Read the model definition and answer for the solid it produces. Units are mm, in the model's axes. Face numbers are marked on the shaded views. A direction names the side the tool comes from. Give positions to 0.01 mm unless a question says otherwise; leave off trailing zeros. Write each loop counter-clockwise with the first axis right and the second up, starting at its lowest first coordinate (ties: lowest second). Pieces come first, ordered by that corner, then holes. Notation, with made-up numbers: (9, 22) -> (42, 22) arc R23 ccw to (42, 61) -> close; hole circle Ø10 at (-13, 39.5). An arc over 180 degrees is marked (long way). Put each result on its own line as item: value. Start each with the question number.
from build123d import *

# Parameters (mm, degrees)
SKETCH1_W           = 130
SKETCH1_H           = 30
BOSS_EXTRUDE1_DEPTH = 5
BOSS_EXTRUDE3_DEPTH = 1.8
SKETCH6_W           = 40
SKETCH6_H           = 25
CUT_EXTRUDE2_DEPTH  = 2
SKETCH5_R           = 1.35
CUT_EXTRUDE3_DEPTH  = 6
SKETCH8_W           = 5
SKETCH8_H           = 30
BOSS_EXTRUDE4_DEPTH = 50
SKETCH9_R           = 10
CUT_EXTRUDE4_DEPTH  = 5
SKETCH10_W          = 30
SKETCH10_H          = 11.1
BOSS_EXTRUDE5_DEPTH = 30
SKETCH11_W          = 3.4
SKETCH11_H          = 30
CUT_EXTRUDE5_DEPTH  = 7
CUT_EXTRUDE6_REACH  = 173.828
SKETCH12_R          = 2.05
CUT_EXTRUDE7_DEPTH  = 5
SKETCH14_W          = 17.3
SKETCH14_H          = 30
CUT_EXTRUDE8_DEPTH  = 2
SKETCH15_W          = 2
SKETCH15_H          = 3
CUT_EXTRUDE9_DEPTH  = 15
FILLET1_START       = -1
FILLET1_DEPTH       = 161
FILLET1_START_2     = 5
FILLET1_2_DEPTH     = 155
FILLET3_R           = 1
FILLET6_R           = 1


with BuildPart() as part:
    # Sketch1 → Boss-Extrude1 (new body)
    with BuildSketch(Plane(origin=(0, 0, 0), x_dir=(1, 0, 0), z_dir=(0, 1, 0))):
        with Locations((65, -15)):
            Rectangle(SKETCH1_W, SKETCH1_H)
    extrude(amount=BOSS_EXTRUDE1_DEPTH)

    # Sketch4 → Boss-Extrude3 (add)
    with BuildSketch(Plane.XZ):
        Polygon((63.1, 25), (66.9, 25), (66.9, 17), (66.9, 16.95), (67.95, 16.95), (74.95, 16.95), (74.95, 13.15), (66.95, 13.15), (66.9, 13.15), (66.9, 12.1), (66.9, 5.1), (63.1, 5.1), (63.1, 13.1), (63.1, 13.15), (62.05, 13.15), (55.05, 13.15), (55.05, 16.95), (63.05, 16.95), (63.1, 16.95), (63.1, 18), align=None)
    extrude(amount=BOSS_EXTRUDE3_DEPTH)

    # Sketch6 → Cut-Extrude2 (cut)
    with BuildSketch(Plane(origin=(0, 5, 0), x_dir=(1, 0, 0), z_dir=(0, 1, 0))):
        with Locations((65, -15)):
            Rectangle(SKETCH6_W, SKETCH6_H)
    extrude(amount=-CUT_EXTRUDE2_DEPTH, mode=Mode.SUBTRACT)

    # Sketch5 → Cut-Extrude3 (cut)
    with BuildSketch(Plane.XZ.offset(1.8)):
        with Locations(Location((65, 23, 0), (0, 0, 270))):
            Circle(SKETCH5_R)
        with Locations(Location((73, 15, 0), (0, 0, 270))):
            Circle(SKETCH5_R)
        with Locations(Location((57, 15, 0), (0, 0, 270))):
            Circle(SKETCH5_R)
        with Locations(Location((65, 7, 0), (0, 0, 270))):
            Circle(SKETCH5_R)
    extrude(amount=-CUT_EXTRUDE3_DEPTH, mode=Mode.SUBTRACT)

    # Sketch8 → Boss-Extrude4 (add)
    with BuildSketch(Plane(origin=(0, 5, 0), x_dir=(1, 0, 0), z_dir=(0, 1, 0))):
        with Locations((2.5, -15)):
            Rectangle(SKETCH8_W, SKETCH8_H)
        with Locations((127.5, -15)):
            Rectangle(SKETCH8_W, SKETCH8_H)
    extrude(amount=BOSS_EXTRUDE4_DEPTH)

    # Sketch9 → Cut-Extrude4 (cut)
    with BuildSketch(Plane(origin=(130, 0, 0), x_dir=(0, 0, -1), z_dir=(1, 0, 0))):
        with Locations((-15, 40)):
            Circle(SKETCH9_R)
    extrude(amount=-CUT_EXTRUDE4_DEPTH, mode=Mode.SUBTRACT)

    # Sketch10 → Boss-Extrude5 (add)
    with BuildSketch(Plane(origin=(130, 0, 0), x_dir=(0, 0, -1), z_dir=(1, 0, 0))):
        with Locations((-15, 13.55)):
            Rectangle(SKETCH10_W, SKETCH10_H)
    extrude(amount=BOSS_EXTRUDE5_DEPTH)

    # Sketch11 → Cut-Extrude5 (cut)
    with BuildSketch(Plane(origin=(0, 19.1, 0), x_dir=(1, 0, 0), z_dir=(0, 1, 0))):
        with Locations((131.7, -15)):
            Rectangle(SKETCH11_W, SKETCH11_H)
        with Locations((152.4, -15)):
            Rectangle(SKETCH11_W, SKETCH11_H)
    extrude(amount=-CUT_EXTRUDE5_DEPTH, mode=Mode.SUBTRACT)

    # Cut-Extrude6: up to this face of the body (flat: up to its plane)
    cut_extrude6_end = Plane(part.part.faces().sort_by_distance((130, 12.623489255, 15))[0])
    # Sketch12 → Cut-Extrude6 (cut, up to the picked face)
    with BuildSketch(Plane(origin=(160, 0, 0), x_dir=(0, 0, -1), z_dir=(1, 0, 0)), mode=Mode.PRIVATE) as cut_extrude6_sk1:
        with Locations((-15, 16)):
            Circle(SKETCH12_R)
    cut_extrude6_tool1 = split(extrude(cut_extrude6_sk1.sketch, amount=-CUT_EXTRUDE6_REACH, mode=Mode.PRIVATE), bisect_by=cut_extrude6_end, keep=Keep.BOTH, mode=Mode.PRIVATE)
    # Sketch12 → Cut-Extrude6 (cut, up to the picked face)
    with BuildSketch(Plane(origin=(160, 0, 0), x_dir=(0, 0, -1), z_dir=(1, 0, 0)), mode=Mode.PRIVATE) as cut_extrude6_sk2:
        with Locations((-21, 16)):
            Circle(SKETCH12_R)
    cut_extrude6_tool2 = split(extrude(cut_extrude6_sk2.sketch, amount=-CUT_EXTRUDE6_REACH, mode=Mode.PRIVATE), bisect_by=cut_extrude6_end, keep=Keep.BOTH, mode=Mode.PRIVATE)
    # Sketch12 → Cut-Extrude6 (cut, up to the picked face)
    with BuildSketch(Plane(origin=(160, 0, 0), x_dir=(0, 0, -1), z_dir=(1, 0, 0)), mode=Mode.PRIVATE) as cut_extrude6_sk3:
        with Locations((-9, 16)):
            Circle(SKETCH12_R)
    cut_extrude6_tool3 = split(extrude(cut_extrude6_sk3.sketch, amount=-CUT_EXTRUDE6_REACH, mode=Mode.PRIVATE), bisect_by=cut_extrude6_end, keep=Keep.BOTH, mode=Mode.PRIVATE)
    add(cut_extrude6_tool1.solids().sort_by(Axis((160, 16, 15), (-1, 0, 0)))[0], mode=Mode.SUBTRACT)
    add(cut_extrude6_tool2.solids().sort_by(Axis((160, 16, 21), (-1, 0, 0)))[0], mode=Mode.SUBTRACT)
    add(cut_extrude6_tool3.solids().sort_by(Axis((160, 16, 9), (-1, 0, 0)))[0], mode=Mode.SUBTRACT)

    # Sketch13 → Cut-Extrude7 (cut)
    with BuildSketch(Plane.ZY):
        with BuildLine():
            Line((9, 40), (9, 55))
            Line((9, 55), (21, 55))
            Line((21, 55), (21, 40))
            ThreePointArc((21, 40), (15, 34), (9, 40))
        make_face()
    extrude(amount=-CUT_EXTRUDE7_DEPTH, mode=Mode.SUBTRACT)

    # Sketch14 → Cut-Extrude8 (cut)
    with BuildSketch(Plane(origin=(0, 19.1, 0), x_dir=(1, 0, 0), z_dir=(0, 1, 0))):
        with Locations((142.05, -15)):
            Rectangle(SKETCH14_W, SKETCH14_H)
    extrude(amount=-CUT_EXTRUDE8_DEPTH, mode=Mode.SUBTRACT)

    # Sketch15 → Cut-Extrude9 (cut)
    with BuildSketch(Plane(origin=(0, 55, 0), x_dir=(1, 0, 0), z_dir=(0, 1, 0))):
        with Locations((2.5, -7.5)):
            Rectangle(SKETCH15_W, SKETCH15_H)
        with Locations((2.5, -22.5)):
            Rectangle(SKETCH15_W, SKETCH15_H)
    extrude(amount=-CUT_EXTRUDE9_DEPTH, mode=Mode.SUBTRACT)

    # Fillet1: read off the stored shape, not the designer's step
    # Fillet1 outline → Fillet1 (cut)
    with BuildSketch(Plane.YZ.offset(FILLET1_START)):
        with BuildLine():
            Line((55, 0), (55, 9))
            ThreePointArc((55, 9), (51.758329561, 2.583801513), (45.050125629, 0))
            Line((45.050125629, 0), (55, 0))
        make_face()
        with BuildLine():
            ThreePointArc((45.050125629, 30), (51.758329561, 27.416198487), (55, 21))
            Line((55, 21), (55, 30))
            Line((55, 30), (45.050125629, 30))
        make_face()
    extrude(amount=FILLET1_DEPTH, mode=Mode.SUBTRACT)

    # Fillet1 2 outline → Fillet1 2 (cut)
    with BuildSketch(Plane.YZ.offset(FILLET1_START_2)):
        with BuildLine():
            ThreePointArc((45, 30), (52.071067812, 27.071067812), (55, 20))
            Line((55, 20), (55, 21))
            ThreePointArc((55, 21), (51.758329561, 27.416198487), (45.050125629, 30))
            Line((45.050125629, 30), (45, 30))
        make_face()
        with BuildLine():
            ThreePointArc((45.050125629, 0), (51.758329561, 2.583801513), (55, 9))
            Line((55, 9), (55, 10))
            ThreePointArc((55, 10), (52.071067812, 2.928932188), (45, 0))
            Line((45, 0), (45.050125629, 0))
        make_face()
    extrude(amount=FILLET1_2_DEPTH, mode=Mode.SUBTRACT)

    # Fillet3
    fillet3_edges = [part.edges().sort_by_distance(p)[0] for p in [
        (4.25, 55, 9),
        (4.25, 55, 21),
    ]]
    fillet(fillet3_edges, radius=FILLET3_R)

    # Fillet6
    fillet6_edges = [part.edges().sort_by_distance(p)[0] for p in [
        (130, 40, 25),
        (125, 40, 25),
    ]]
    fillet(fillet6_edges, radius=FILLET6_R)


solid = part.part
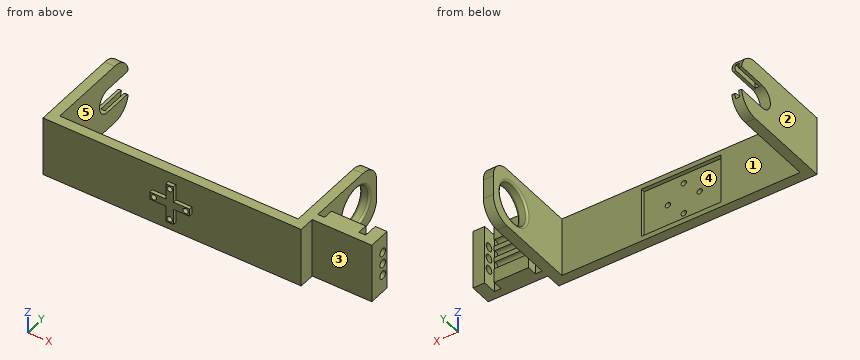
1) A cutting plane is placed at B-B on y = 46.5. State how many separate pieces and enclosed holes the cut face has, and give its area (3 significant figures).
2) For a pull along X with two mould halves and no side action, classify the marked faces 1, 2 and 3 as pulls with the +X half, pulls with the -X half, needs draft (parallel to the pull), parting line crosses it, or undercut.
3) For the marked faces 4 and 5, determine the directions among +Z, -Z, +X, -X, +Y, -Y from which every point of the face is accessible in a straight line to the end or side of a thin tool.
4) Straight lines are drawn through the part: line 1 (X direction, y = 0.7, z = 15); line 2 (Z direction, x = 143, y = 16); line 3 (X direction, y = 9, z = 21). For each, find the intervals that lie inside material, in ascending order. Write a range as [from, to].
5) A cutting plane is placed at A-A on x = 147.5. Give the vertices of the cut face in (y, z).
6) Each of these flat-tipped pins is pushed along its axis until it touches: pin 1 Ø7.5 at (x, z) = (61.5, 19.5) entering from +Y; pin 2 Ø1 at (x, z) = (102, 22) entering from +Y; pin 3 Ø0.5 at (y, z) = (-1, 15.5) entering from -X. Where does it stop, or does it pass through?
7) A cutting plane is placed at C-C on x = 88. Give the vertices of the cut face in (y, z), and give its area (3 significant figures).
Results found:
1. separate pieces: 4
1. enclosed holes: 0
1. area: 149 mm²
2. face 1: undercut
2. face 2: pulls with the -X half
2. face 3: needs draft
3. face 4: +Y
3. face 5: +Z, -Z, +Y
4. line 1: x = [0, 55.65], [58.35, 71.65], [74.35, 130]
4. line 2: z = [0, 6.95], [11.05, 12.95], [17.05, 18.95], [23.05, 30]
4. line 3: x = [0, 5], [125, 160]
5. outline: (8, 0) -> (17.1, 0) -> (17.1, 7.27) arc R2.05 cw (long way) to (17.1, 10.73) -> (17.1, 13.27) arc R2.05 cw (long way) to (17.1, 16.73) -> (17.1, 19.27) arc R2.05 cw (long way) to (17.1, 22.73) -> (17.1, 30) -> (8, 30) -> close
6. pin 1: stops at y = 3
6. pin 2: stops at y = 5
6. pin 3: stops at x = 55.05
7. outline: (0, 0) -> (5, 0) -> (5, 30) -> (0, 30) -> close
7. area: 150 mm²
